Autodesk Inventor part; units mm, degrees
ref_plane "YZ Plane" through (0, 0, 0) normal (1, 0, 0) x (0, 1, 0)
ref_plane "XZ Plane" through (0, 0, 0) normal (0, 1, 0) x (-1, 0, 0)
ref_plane "XY Plane" through (0, 0, 0) normal (0, 0, 1) x (1, 0, 0)
sketch "Sketch1" plane through (0, 0, 0) normal (0, 0, 1) x (1, 0, 0)
  circle A0 centre (12.05, 22.55) radius 1.45
  circle A1 centre (-12.05, 22.55) radius 1.45
  circle A2 centre (-12.05, -22.55) radius 1.45
  circle A3 centre (12.05, -22.55) radius 1.45
  line L0 (15, -25) -> (-15, -25)
  line L1 (15, 25) -> (15, -25)
  line L2 (-15, 25) -> (15, 25)
  line L3 (-15, -25) -> (-15, 25)
  point P0 (0, 0)
extrude "Extrusion1" add sketch "Sketch1" along normal blind 1
sketch "Sketch2" plane through (0, 0, 1) normal (0, 0, 1) x (1, 0, 0)
  line L0 (15, 25) -> (-15, 25)
  line L1 (-15, 25) -> (-15, -25)
  line L2 (-15, -25) -> (15, -25)
  line L3 (15, -25) -> (15, 25)
  circle A0 centre (12.05, -22.55) radius 1.45
  circle A1 centre (-12.05, -22.55) radius 1.45
  circle A2 centre (-12.05, 22.55) radius 1.45
  circle A3 centre (12.05, 22.55) radius 1.45
  point P0 (0, 0)
extrude "Extrusion2" add sketch "Sketch2" along normal blind 5 and the other way blind 1 contours A0 | A1 | A2 | A3
chamfer "Chamfer1" distance 0.8 angle 45 4 edges at (-13.5, -22.55, 6) (-13.5, 22.55, 6) (10.6, 22.55, 6) (10.6, -22.55, 6)
properties part number "buck_holes_check"
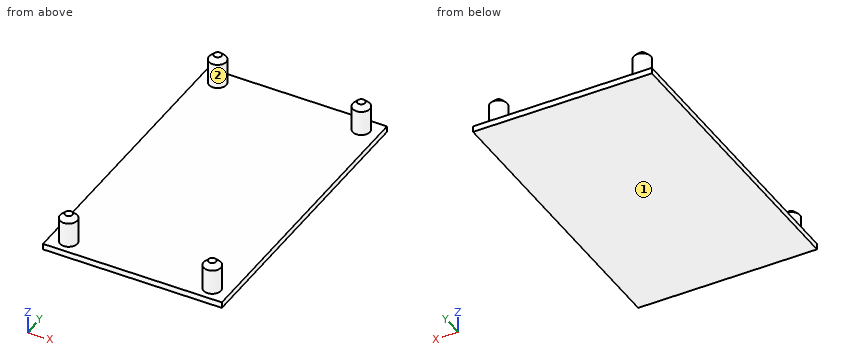
For this review, take the finished solid that the model builds, in its own axes (mm). Face numbers are marked on the shaded views. Give positions to 0.01 mm unless a question says otherwise; leave off trailing zeros. Loops run counter-clockwise (first coordinate to the right, second up) from the corner with the lowest first, then second, coordinate; pieces in that order, holes last. Notation, with made-up numbers: M 55.5,18 L 92.5,18 A20 cw 92.5,46 Z; hole C -14.5,59 d10. An arc over 180 degrees is marked long. One line per item, written item: value. Start each with the question number.
Q1. Add section D-D (x = -1.25). Give the boundary of the cut face in (y, z), and give its area (3 significant figures).
Q2. Add section C-C (z = 2.5). Give the boundary of the cut face in (x, y).
Q3. For L1, parallel to Z at x = -4, y = 11, list the stretches that pass through material, from the lowest coordinate up.
Q4. Clearance check with a flat-ended pin moving along its axis: pin 1 Ø9 at (x, y) = (3, 1) entering from +Z. State where the tip first meets the part, or that it passes through.
Q5. Add section B-B (y = 22.55). Give the boundary of the cut face in (x, z), and give its area (3 significant figures).
Q6. Add section A-A (x = 12.05). Give the boundary of the cut face in (y, z), and give its area (3 significant figures).
Q7. Draft analysis for pull direction X (two halves, no side actions). For the marked faces 1 and 2, state which applies: released by +X, released by -X, zero draft, split by the parting line, or undercut.
Reply:
1. outline: M -25,0 L 25,0 L 25,1 L -25,1 Z
1. area: 50.0 mm²
2. outline: C -12.05,-22.55 d2.9; C -12.05,22.55 d2.9; C 12.05,-22.55 d2.9; C 12.05,22.55 d2.9
3. L1: 0 to 1
4. pin 1: z = 1
5. outline: M -15,0 L 15,0 L 15,1 L 13.5,1 L 13.5,5.2 L 12.7,6 L 11.4,6 L 10.6,5.2 L 10.6,1 L -10.6,1 L -10.6,5.2 L -11.4,6 L -12.7,6 L -13.5,5.2 L -13.5,1 L -15,1 Z
5. area: 57.7 mm²
6. outline: M -25,0 L 25,0 L 25,1 L 24,1 L 24,5.2 L 23.2,6 L 21.9,6 L 21.1,5.2 L 21.1,1 L -21.1,1 L -21.1,5.2 L -21.9,6 L -23.2,6 L -24,5.2 L -24,1 L -25,1 Z
6. area: 77.7 mm²
7. face 1: zero draft
7. face 2: undercut
